Source: CAD feature listing. Evaluate the final solid. Frame: model axes, mm. Face numbers are marked on the shaded views. A direction names the side the tool comes from. Give positions to 0.01 mm unless a question says otherwise; leave off trailing zeros. Loops run counter-clockwise (first coordinate to the right, second up) from the corner with the lowest first, then second, coordinate; pieces in that order, holes last. Notation, with made-up numbers: (74, 30) -> (103, 30) arc R9 ccw to (103, 41) -> close; hole circle Ø8 at (0, 10). An arc over 180 degrees is marked (long way). Return JSON: item names as keys, results as strings. Group by question number.
(1) Cut plane B-B on x = -4. Return loops of the section in (y, z).
(2) Cut plane C-C on z = 27. Return loops of the section in (x, y).
(3) Cut plane D-D on x = 0. Return loops of the section in (y, z), then the cut area to 3 significant figures.
(4) Access query for the marked faces 5, 6, 7, 8 and 9. Directions: +Z, -Z, +X, -X, +Y, -Y. A direction counts if a zero-diameter tool reaches every point of the face in a straight line with its end or side. Return the directions, or none.
(5) Cut plane A-A on y = 5. Return loops of the section in (x, z), then the cut area to 3 significant figures.
(6) Draft query along Z for the marked faces 1, 2, 3 and 4. Return one class per face: released by +Z, released by -Z, zero draft, split by the parting line, or undercut.
(7) Pin query (flat end, axial travel): pin 1 (1.5 mm diameter, centred on x = 11.5, y = -31, fed in from -Z); pin 2 (16.5 mm diameter, centred on x = 4, z = 6, fed in from -Y); pin 3 (13 mm diameter, centred on x = 0, z = 25, fed in from +Y). Return the tip coordinate at first contact, or that it passes through.
(8) Ray query, line 1 (Z direction, x = 0, y = 10.5); line 2 (Y direction, x = 0, z = 24.5); line 3 (Z direction, x = 0.5, y = -3.5). Return the intervals inside material, ascending. Write a range as from..to.
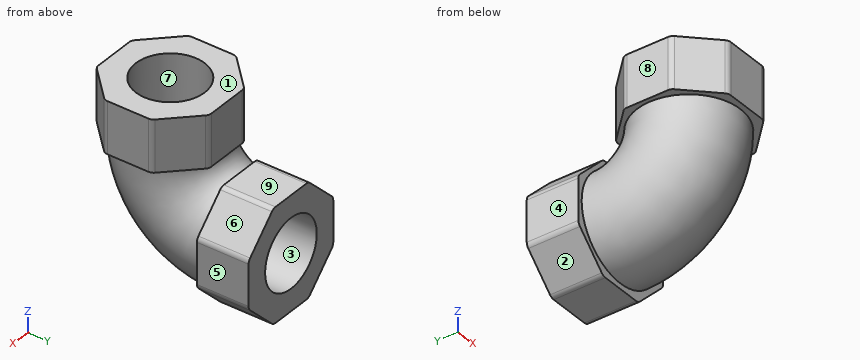
```python
from build123d import *

# Parameters (mm, degrees)
F0_R     = 15
F0_R_2   = 10
F3_R     = 10
F4_DEPTH = 15
F5_R     = 15
F5_R_2   = 10
F6_DEPTH = 15


with BuildPart() as f2:
    # F2: sweep along a path in F1
    with BuildLine(Plane.YZ) as f2_path:
        ThreePointArc((-20, 20), (-14.1421356237, 5.8578643763), (0, 0))
    # F0 (on Front) → F2 (sweep)
    with BuildSketch(Plane.XZ):
        with Locations((-0.1311794548, 0.1967689097)):
            Circle(F0_R)
        Circle(F0_R_2, mode=Mode.SUBTRACT)
    sweep(path=f2_path.line)

    # F3 (on Front) → F4 (join)
    with BuildSketch(Plane.XZ):
        with BuildLine():
            Line((5.9544622317, 16.3753434763), (-5.9544622317, 16.3753434763))
            ThreePointArc((-5.9544622317, 16.3753434763), (-6.7198290964, 16.2231025413), (-7.368675794, 15.7895570387))
            Line((-7.368675794, 15.7895570387), (-15.7895570387, 7.368675794))
            ThreePointArc((-15.7895570387, 7.368675794), (-16.2231025413, 6.7198290964), (-16.3753434763, 5.9544622317))
            Line((-16.3753434763, 5.9544622317), (-16.3753434763, -5.9544622317))
            ThreePointArc((-16.3753434763, -5.9544622317), (-16.2231025413, -6.7198290964), (-15.7895570387, -7.368675794))
            Line((-15.7895570387, -7.368675794), (-7.368675794, -15.7895570387))
            ThreePointArc((-7.368675794, -15.7895570387), (-6.7198290964, -16.2231025413), (-5.9544622317, -16.3753434763))
            Line((-5.9544622317, -16.3753434763), (5.9544622317, -16.3753434763))
            ThreePointArc((5.9544622317, -16.3753434763), (6.7198290964, -16.2231025413), (7.368675794, -15.7895570387))
            Line((7.368675794, -15.7895570387), (15.7895570387, -7.368675794))
            ThreePointArc((15.7895570387, -7.368675794), (16.2231025413, -6.7198290964), (16.3753434763, -5.9544622317))
            Line((16.3753434763, -5.9544622317), (16.3753434763, 5.9544622317))
            ThreePointArc((16.3753434763, 5.9544622317), (16.2231025413, 6.7198290964), (15.7895570387, 7.368675794))
            Line((15.7895570387, 7.368675794), (7.368675794, 15.7895570387))
            ThreePointArc((7.368675794, 15.7895570387), (6.7198290964, 16.2231025413), (5.9544622317, 16.3753434763))
        make_face()
        Circle(F3_R, mode=Mode.SUBTRACT)
    extrude(amount=-F4_DEPTH)

    # F5 (on face) → F6 (join)
    with BuildSketch(Plane.XY.offset(20)):
        with BuildLine():
            Line((5.9544622317, -3.6246565237), (-5.9544622317, -3.6246565237))
            ThreePointArc((-5.9544622317, -3.6246565237), (-6.7198290964, -3.7768974587), (-7.368675794, -4.2104429613))
            Line((-7.368675794, -4.2104429613), (-15.7895570387, -12.631324206))
            ThreePointArc((-15.7895570387, -12.631324206), (-16.2231025413, -13.2801709036), (-16.3753434763, -14.0455377683))
            Line((-16.3753434763, -14.0455377683), (-16.3753434763, -25.9544622317))
            ThreePointArc((-16.3753434763, -25.9544622317), (-16.2231025413, -26.7198290964), (-15.7895570387, -27.368675794))
            Line((-15.7895570387, -27.368675794), (-7.368675794, -35.7895570387))
            ThreePointArc((-7.368675794, -35.7895570387), (-6.7198290964, -36.2231025413), (-5.9544622317, -36.3753434763))
            Line((-5.9544622317, -36.3753434763), (5.9544622317, -36.3753434763))
            ThreePointArc((5.9544622317, -36.3753434763), (6.7198290964, -36.2231025413), (7.368675794, -35.7895570387))
            Line((7.368675794, -35.7895570387), (15.7895570387, -27.368675794))
            ThreePointArc((15.7895570387, -27.368675794), (16.2231025413, -26.7198290964), (16.3753434763, -25.9544622317))
            Line((16.3753434763, -25.9544622317), (16.3753434763, -14.0455377683))
            ThreePointArc((16.3753434763, -14.0455377683), (16.2231025413, -13.2801709036), (15.7895570387, -12.631324206))
            Line((15.7895570387, -12.631324206), (7.368675794, -4.2104429613))
            ThreePointArc((7.368675794, -4.2104429613), (6.7198290964, -3.7768974587), (5.9544622317, -3.6246565237))
        make_face()
        with Locations((-0.1311794548, -19.8032310903)):
            Circle(F5_R, mode=Mode.SUBTRACT)
        with Locations((-0.1311794548, -19.8032310903)):
            Circle(F5_R)
        with Locations((0, -20)):
            Circle(F5_R_2, mode=Mode.SUBTRACT)
    extrude(amount=F6_DEPTH)


solid = f2.part
```
Answers:
{
 "1": {"outline": "(-36.38, 20) -> (-34.3, 20) arc R34.3 ccw to (0, -14.3) -> (0, -16.38) -> (15, -16.38) -> (15, -9.17) -> (0, -9.17) arc R29.17 cw to (-29.17, 20) -> (-29.17, 35) -> (-36.38, 35) -> close; (-10.83, 20) arc R10.83 ccw to (0, 9.17) -> (15, 9.17) -> (15, 16.38) -> (0, 16.38) -> (0, 14.69) arc R5.31 cw to (-5.31, 20) -> (-3.62, 20) -> (-3.62, 35) -> (-10.83, 35) -> close"},
 "2": {"outline": "(-16.38, -25.95) arc R2 ccw to (-15.79, -27.37) -> (-7.37, -35.79) arc R2 ccw to (-5.95, -36.38) -> (5.95, -36.38) arc R2 ccw to (7.37, -35.79) -> (15.79, -27.37) arc R2 ccw to (16.38, -25.95) -> (16.38, -14.05) arc R2 ccw to (15.79, -12.63) -> (7.37, -4.21) arc R2 ccw to (5.95, -3.62) -> (-5.95, -3.62) arc R2 ccw to (-7.37, -4.21) -> (-15.79, -12.63) arc R2 ccw to (-16.38, -14.05) -> close; hole circle Ø20 at (0, -20)"},
 "3": {"outline": "(-36.38, 20) -> (-34.8, 20) arc R34.8 ccw to (0, -14.8) -> (0, -16.38) -> (15, -16.38) -> (15, -10) -> (0, -10) arc R30 cw to (-30, 20) -> (-30, 35) -> (-36.38, 35) -> close; (-10, 20) arc R10 ccw to (0, 10) -> (15, 10) -> (15, 16.38) -> (0, 16.38) -> (0, 15.2) arc R4.8 cw to (-4.8, 20) -> (-3.62, 20) -> (-3.62, 35) -> (-10, 35) -> close", "area": "687 mm²"},
 "4": {"face 5": "+Z, -Z, +X, +Y, -Y", "face 6": "+Z, +X, +Y", "face 7": "+Z", "face 8": "+Z, -Z, -X, +Y, -Y", "face 9": "+Z, +X, -X, +Y"},
 "5": {"outline": "(-16.38, -5.95) arc R2 ccw to (-15.79, -7.37) -> (-7.37, -15.79) arc R2 ccw to (-5.95, -16.38) -> (5.95, -16.38) arc R2 ccw to (7.37, -15.79) -> (15.79, -7.37) arc R2 ccw to (16.38, -5.95) -> (16.38, 5.95) arc R2 ccw to (15.79, 7.37) -> (7.37, 15.79) arc R2 ccw to (5.95, 16.38) -> (-5.95, 16.38) arc R2 ccw to (-7.37, 15.79) -> (-15.79, 7.37) arc R2 ccw to (-16.38, 5.95) -> close; hole circle Ø20 at (0, 0)", "area": "574 mm²"},
 "6": {"face 1": "released by +Z", "face 2": "released by -Z", "face 3": "undercut", "face 4": "zero draft"},
 "7": {"pin 1": "z = 20", "pin 2": "y = -34.18", "pin 3": "y = -3.62"},
 "8": {"line 1": "-16.38..-10, 10..16.38", "line 2": "-36.38..-30, -10..-3.62", "line 3": "-14.61..-9.78, 10.62..16.69"}
}
